```python
from build123d import *

# Parameters (mm, degrees)
SKETCH1_W           = 60
SKETCH1_H           = 105
BOSS_EXTRUDE4_DEPTH = 6
BOSS_EXTRUDE5_DEPTH = 25
SKETCH1_15_R        = 2
CUT_EXTRUDE1_DEPTH  = 25
SKETCH1_16_R        = 4
SKETCH1_16_R_2      = 2
CUT_EXTRUDE2_DEPTH  = 25
SKETCH1_18_R        = 4
SKETCH1_18_R_2      = 2
BOSS_EXTRUDE7_DEPTH = 3
FILLET1_R           = 10
SKETCH2_W           = 5
SKETCH2_H           = 24
CUT_EXTRUDE3_DEPTH  = 19


with BuildPart() as part:
    # Sketch1 → Boss-Extrude4 (new body)
    with BuildSketch(Plane.XY):
        with Locations((30, 52.5)):
            Rectangle(SKETCH1_W, SKETCH1_H)
    extrude(amount=BOSS_EXTRUDE4_DEPTH)

    # Sketch1<12> → Boss-Extrude5 (add)
    with BuildSketch(Plane.XY):
        Polygon((5, 5), (5, 105), (0, 105), (0, 0), (60, 0), (60, 5), align=None)
    extrude(amount=BOSS_EXTRUDE5_DEPTH)

    # Sketch1<15> → Cut-Extrude1 (cut)
    with BuildSketch(Plane.XY):
        with Locations((50, 95)):
            Circle(SKETCH1_15_R)
        with Locations((15, 95)):
            Circle(SKETCH1_15_R)
    extrude(amount=CUT_EXTRUDE1_DEPTH, mode=Mode.SUBTRACT)

    # Sketch1<16> → Cut-Extrude2 (cut)
    # profile 1 of 2: a face of its own
    with BuildSketch(Plane.XY):
        with Locations((50, 95)):
            Circle(SKETCH1_16_R)
        with Locations((50, 95)):
            Circle(SKETCH1_16_R_2, mode=Mode.SUBTRACT)
    # profile 2 of 2: a face of its own
    with BuildSketch(Plane.XY):
        with Locations((15, 95)):
            Circle(SKETCH1_16_R)
        with Locations((15, 95)):
            Circle(SKETCH1_16_R_2, mode=Mode.SUBTRACT)
    extrude(amount=CUT_EXTRUDE2_DEPTH, mode=Mode.SUBTRACT)

    # Sketch1<18> → Boss-Extrude7 (add)
    # profile 1 of 2: a face of its own
    with BuildSketch(Plane.XY):
        with Locations((50, 95)):
            Circle(SKETCH1_18_R)
        with Locations((50, 95)):
            Circle(SKETCH1_18_R_2, mode=Mode.SUBTRACT)
    # profile 2 of 2: a face of its own
    with BuildSketch(Plane.XY):
        with Locations((15, 95)):
            Circle(SKETCH1_18_R)
        with Locations((15, 95)):
            Circle(SKETCH1_18_R_2, mode=Mode.SUBTRACT)
    extrude(amount=BOSS_EXTRUDE7_DEPTH)

    # Fillet1
    fillet1_edges = [part.edges().sort_by_distance(p)[0] for p in [
        (60, 0, 12.5),
        (0, 105, 12.5),
        (0, 0, 12.5),
    ]]
    fillet(fillet1_edges, radius=FILLET1_R)

    # Sketch2 → Cut-Extrude3 (cut)
    with BuildSketch(Plane.XY.offset(25)):
        with Locations((2.5, 41)):
            Rectangle(SKETCH2_W, SKETCH2_H)
    extrude(amount=-CUT_EXTRUDE3_DEPTH, mode=Mode.SUBTRACT)


solid = part.part
```
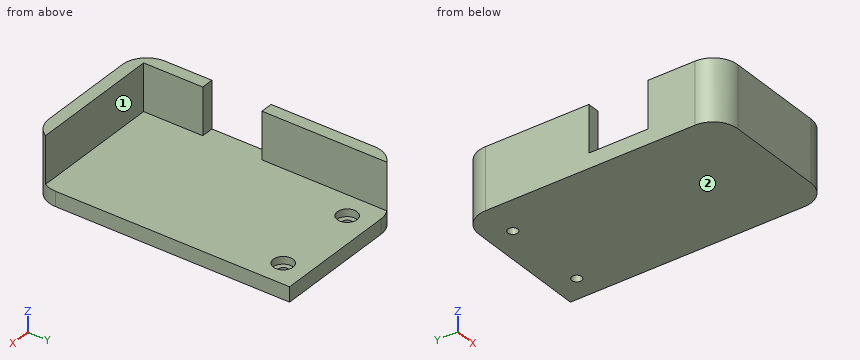
CAD build for the part. Positions are in the model's coordinates, mm. Face numbers are marked on the shaded views. A direction names the side the tool comes from. Give positions to 0.01 mm unless a question says otherwise; leave off trailing zeros. Order: outer loops, then holes, each group sorted by start corner. A loop starts at its lowest first (then second) coordinate and runs counter-clockwise, first axis right, second up.
(1) Tool access for the marked faces 1 and 2: list every direction of +Z, -Z, +X, -X, +Y, -Y with a clear straight run to the whole face (end or side of a thin tool).
(2) Drill centre lines: L1, parallel to Y at x = 15, z = 2.1; L2, parallel to Y at x = 50, z = 4.15; L3, parallel to Z at x = 28, y = 58.5. Where is each one in solid material? Low to high.
(3) Flat gauge pins, fed straight in: pin 1 (5.5 mm diameter, centred on y = 88, z = 17.5, fed in from +X); pin 2 (9 mm diameter, centred on x = 48.5, y = 96.5, fed in from +Z); pin 3 (13 mm diameter, centred on x = 50, y = 95, fed in from -Z); pin 4 (2.5 mm diameter, centred on x = 2.5, z = 14.5, fed in from +Y). Where does each tip first touch, or does it go through?
(4) Saw through at A-A, the plane z = 15.5. Give the cut face in (x, y), then the cut area to 3 significant figures.
(5) Saw through at D-D, the plane y = 66. Give the cut face in (x, z), then the cut area to 3 significant figures.
(6) Saw through at C-C, the plane z = 4.25. Give the cut face in (x, y).
(7) Saw through at B-B, the plane x = 15. Give the cut face in (y, z), then the cut area to 3 significant figures.
Results found:
1. face 1: +Z, +X, +Y
1. face 2: -Z, +X, -X, +Y, -Y
2. L1: y = 0 to 93, 97 to 105
2. L2: y = 0 to 91, 99 to 105
2. L3: z = 0 to 6
3. pin 1: stops at x = 5
3. pin 2: stops at z = 6
3. pin 3: stops at z = 0
3. pin 4: stops at y = 102.81
4. outline: (0, 10) arc R10 ccw to (10, 0) - (50, 0) arc R10 ccw to (58.66, 5) - (5, 5) - (5, 29) - (0, 29) - close; (0, 53) - (5, 53) - (5, 103.66) arc R10 ccw to (0, 95) - close
4. area: 620 mm2
5. outline: (0, 0) - (60, 0) - (60, 6) - (5, 6) - (5, 25) - (0, 25) - close
5. area: 455 mm2
6. outline: (0, 10) arc R10 ccw to (10, 0) - (50, 0) arc R10 ccw to (60, 10) - (60, 105) - (10, 105) arc R10 ccw to (0, 95) - close; hole circle Ø8 at (15, 95); hole circle Ø8 at (50, 95)
7. outline: (0, 0) - (93, 0) - (93, 3) - (91, 3) - (91, 6) - (5, 6) - (5, 25) - (0, 25) - close; (97, 0) - (105, 0) - (105, 6) - (99, 6) - (99, 3) - (97, 3) - close
7. area: 689 mm2
